```python
from build123d import *

# Parameters (mm, degrees)
SKETCH1_R           = 38.0365
SKETCH1_R_2         = 6.5024
SKETCH1_R_3         = 7.62
BOSS_EXTRUDE1_DEPTH = 9.525
SKETCH2_R           = 38.0365
SKETCH2_R_2         = 33.02
BOSS_EXTRUDE2_DEPTH = 63.5
SKETCH3_R           = 12.7
SKETCH3_R_2         = 6.5024
BOSS_EXTRUDE3_DEPTH = 15.875
CHAMFER1_SIZE       = 6.35
CHAMFER1_SIZE2      = 2.54
SKETCH4_R           = 12.7
BOSS_EXTRUDE4_DEPTH = 6.35
FILLET1_R           = 2.54


with BuildPart() as part:
    # Sketch1 → Boss-Extrude1 (new body)
    with BuildSketch(Plane(origin=(0, 0, 0), x_dir=(1, 0, 0), z_dir=(0, 1, 0))):
        Circle(SKETCH1_R)
        Circle(SKETCH1_R_2, mode=Mode.SUBTRACT)
        with Locations((0, 22.86)):
            Circle(SKETCH1_R_3, mode=Mode.SUBTRACT)
        with Locations((21.741151963, 7.064128491)):
            Circle(SKETCH1_R_3, mode=Mode.SUBTRACT)
        with Locations((13.436770867, -18.494128491)):
            Circle(SKETCH1_R_3, mode=Mode.SUBTRACT)
        with Locations((-13.436770867, -18.494128491)):
            Circle(SKETCH1_R_3, mode=Mode.SUBTRACT)
        with Locations((-21.741151963, 7.064128491)):
            Circle(SKETCH1_R_3, mode=Mode.SUBTRACT)
    extrude(amount=BOSS_EXTRUDE1_DEPTH)

    # Sketch2 → Boss-Extrude2 (add)
    with BuildSketch(Plane(origin=(0, 9.525, 0), x_dir=(1, 0, 0), z_dir=(0, 1, 0))):
        Circle(SKETCH2_R)
        Circle(SKETCH2_R_2, mode=Mode.SUBTRACT)
    extrude(amount=BOSS_EXTRUDE2_DEPTH)

    # Sketch3 → Boss-Extrude3 (add)
    with BuildSketch(Plane(origin=(0, 9.525, 0), x_dir=(1, 0, 0), z_dir=(0, 1, 0))):
        Circle(SKETCH3_R)
        Circle(SKETCH3_R_2, mode=Mode.SUBTRACT)
    extrude(amount=BOSS_EXTRUDE3_DEPTH)

    # Chamfer1
    chamfer1_edges = [part.edges().sort_by_distance(p)[0] for p in [
        (-38.0365, 73.025, 0),
    ]]
    chamfer1_side = [part.faces().sort_by_distance(p)[0] for p in [
        (-38.0365, 36.5125, 0),
    ]]
    chamfer(chamfer1_edges, length=CHAMFER1_SIZE, length2=CHAMFER1_SIZE2, reference=chamfer1_side[0])

    # Sketch4 → Boss-Extrude4 (add)
    with BuildSketch(Plane(origin=(0, 25.4, 0), x_dir=(1, 0, 0), z_dir=(0, 1, 0))):
        Circle(SKETCH4_R)
    extrude(amount=BOSS_EXTRUDE4_DEPTH)

    # Fillet1
    fillet1_edges = [part.edges().sort_by_distance(p)[0] for p in [
        (-12.7, 31.75, 0),
    ]]
    fillet(fillet1_edges, radius=FILLET1_R)


solid = part.part
```
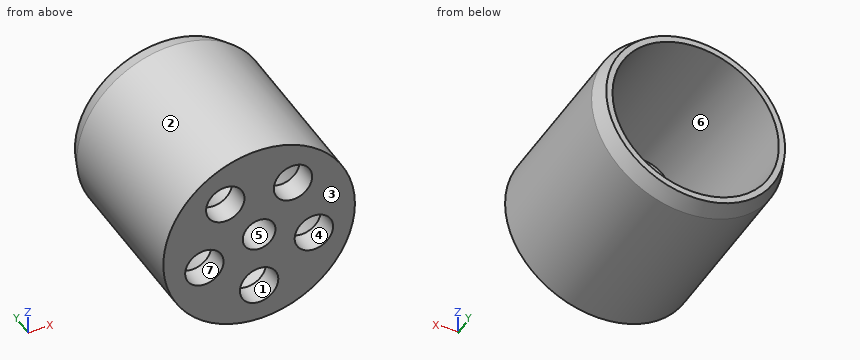
Design review of the part built by this model. Coordinates are the model's own, in mm. Face numbers are marked on the shaded views. A direction names the side the tool comes from. Give positions to 0.01 mm unless a question says otherwise; leave off trailing zeros. Order: outer loops, then holes, each group sorted by start corner. A loop starts at its lowest first (then second) coordinate and runs counter-clockwise, first axis right, second up. Notation, with made-up numbers: (-3.5, 71) -> (24.5, 71) arc R31 ccw to (24.5, 104) -> close; hole circle Ø5 at (13, -3.5). An arc over 180 degrees is marked (long way). Write item = value, one per line. Start each with the question number.
(1) To check wall thickness, follow line 1 along Z through (x, y) = (-0.5, 10.5); line 2 along X through (y, z) = (25.5, -4); line 3 along Z through (x, y) = (6, 63). State the ranges of each line that lie inside material, in increasing order.
(2) We need section B-B on y = 15. Write out the cut boundary in (x, z), plus the area to 3 significant figures.
(3) Mouldability with a two-part tool opening along X and no side actions: class the marked faces 1, 2, 3 and 4 as +X half, -X half, draft (parallel to the pull), parting line (faces both ways), or undercut.
(4) We need section D-D on x = 17. State how many separate pieces and enclosed holes the cut face has, plus the area to 3 significant figures.
(5) We need section C-C on y = 35.5. Write out the cut boundary in (x, z), plus the area to 3 significant figures.
(6) For pin 1 (11.5 mm diameter, centred on x = 0, z = 0, fed in from +Y); pin 2 (12 mm diameter, centred on y = 17.5, z = 10.5, fed in from -X); pin 3 (1 mm diameter, centred on y = 7.5, z = -5.5, fed in from -X); pin 4 (8 mm diameter, centred on x = 20, z = -9, fed in from +Y), all flat-tipped, find the tip position at first contact; note any pin that passes through.
(7) For the marked faces 5, 6 and 7, list the 3-axis set-ups (+Z, -Z, +X, -X, +Y, -Y) from which the entire face can be reached by the end or side of a thin tool; tool diameter is ignored.
Numbers:
q1.line_1 = -38.03 to -33.02, -12.69 to -6.48, 6.48 to 12.69, 33.02 to 38.03
q1.line_2 = -37.83 to -32.78, -12.05 to 12.05, 32.78 to 37.83
q1.line_3 = -37.56 to -32.47, 32.47 to 37.56
q2.outline = circle Ø76.07 at (0, 0); circle Ø25.4 at (0, 0); hole circle Ø66.04 at (0, 0); hole circle Ø13 at (0, 0)
q2.area = 1,490 mm^2
q3.face_1 = undercut
q3.face_2 = parting line
q3.face_3 = draft
q3.face_4 = undercut
q4.separate_pieces = 3
q4.enclosed_holes = 0
q4.area = 1,110 mm^2
q5.outline = circle Ø76.07 at (0, 0); hole circle Ø66.04 at (0, 0)
q5.area = 1,120 mm^2
q6.pin_1 = 31.75
q6.pin_2 = -37.77
q6.pin_3 = -37.71
q6.pin_4 = through
q7.face_5 = -Y
q7.face_6 = +Y
q7.face_7 = +Y, -Y
